from build123d import *

# Parameters (mm, degrees)
BOSS_EXTRUDE1_REACH = 15.24
SKETCH2_R           = 4.7625


with BuildPart() as part:
    # Sketch1 → Revolve1 (revolve)
    with BuildSketch(Plane(origin=(0, 0, 0), x_dir=(0, 0, -1), z_dir=(1, 0, 0)), mode=Mode.PRIVATE) as revolve1_sk:
        Polygon((0, 4.7625), (-7.1628, 4.7625), (-7.1628, 5.55625), (-3.90525, 5.55625), (-1.5875, 7.874), (0, 7.874), align=None)
    revolve(revolve1_sk.sketch.rotate(Axis((0, 0, 0), (0, 0, 1)), 90), axis=Axis((0, 0, 0), (0, 0, 1)))

    # Boss-Extrude1: up to this cone (the profile starts outside it)
    boss_extrude1_end = Plane(origin=(0, 0, 7.1628), z_dir=(0, 0, -1)).offset(-2.298699) * Cone(1e-06, 20.3374, 20.337399, align=(Align.CENTER, Align.CENTER, Align.MIN), mode=Mode.PRIVATE)
    # Sketch2 → Boss-Extrude1 (add, up to the surface)
    with BuildSketch(Plane.XY.offset(7.1628), mode=Mode.PRIVATE) as boss_extrude1_sk1:
        Polygon((-3.207902433, 5.55625), (-6.415804866, 0), (-3.207902433, -5.55625), (3.207902433, -5.55625), (6.415804866, 0), (3.207902433, 5.55625), align=None)
        with Locations(Location((0, 0, 0), (0, 0, 180))):
            Circle(SKETCH2_R, mode=Mode.SUBTRACT)
    boss_extrude1_tool1 = extrude(boss_extrude1_sk1.sketch, amount=-BOSS_EXTRUDE1_REACH, mode=Mode.PRIVATE) - boss_extrude1_end
    add(boss_extrude1_tool1.solids().sort_by_distance((-4.664849, 2.693252, 7.1628))[0])


solid = part.part
Model file for the job. Use its own axes, mm. A direction names the side the tool comes from. Give positions to 0.01 mm unless a question says otherwise; leave off trailing zeros. Loops run counter-clockwise (first coordinate to the right, second up) from the corner with the lowest first, then second, coordinate; pieces in that order, holes last.
1) Wall check: line 1 (Y direction, x = -3.25, z = 2.25); line 2 (Y direction, x = 0, z = 2.5); line 3 (X direction, y = -3.25, z = 4.5). Give the ranges that are in metal, low to high.
2) Saw through at C-C (z = 0.75). Write the cut outline in (x, y) (1 decimal), plus the area to 3 significant figures.
3) Pull direction Y, two halves, no side cores. Call faces 1 (the flat face through (4.8, -2.8, 5.6)), 2 (the flat face through (0, 5.556, 6)), 3 (the cylindrical face through (1.03, 4.65, 3.63)): +Y half, -Y half, draft (parallel to the pull), parting line (faces both ways), or undercut.
4) Tool access for faces 4 (the flat face through (-4.834, -2.739, 5.591)), 5 (the flat face through (4.834, 2.739, 5.591)), 6 (the flat face through (-4.8, 2.8, 5.6)): list every direction of +Z, -Z, +X, -X, +Y, -Y with a clear straight run to the whole face (end or side of a thin tool).
5) Saw through at B-B (x = 0). Write the cut outline in (y, z).
6) Flat gauge pins, fed straight in: pin 1 Ø1 at (x, z) = (-2, 3) entering from -Y; pin 2 Ø3.5 at (x, z) = (-1.5, 5) entering from -Y; pin 3 Ø1 at (x, z) = (-5, 2) entering from -Y. Where does each tip first touch, or does it go through?
7) Saw through at A-A (z = 4.75). Write the cut outline in (x, y) (1 decimal), plus the area to 3 significant figures.
Answer block:
1. line 1: y = -6.44 to -3.48, 3.48 to 6.44
1. line 2: y = -6.96 to -4.76, 4.76 to 6.96
1. line 3: x = -4.54 to -3.48, 3.48 to 4.54
2. outline: circle Ø15.7 at (0, 0); hole circle Ø9.5 at (0, 0)
2. area: 124 mm2
3. face 1: -Y half
3. face 2: +Y half
3. face 3: undercut
4. face 4: +Z, -X, -Y
4. face 5: +Z, +X, +Y
4. face 6: +Z, -X, +Y
5. outline: (-7.87, 0) - (-4.76, 0) - (-4.76, 7.16) - (-5.56, 7.16) - (-5.56, 3.91) - (-7.87, 1.59) - close; (4.76, 0) - (7.87, 0) - (7.87, 1.59) - (5.56, 3.91) - (5.56, 7.16) - (4.76, 7.16) - close
6. pin 1: stops at y = -6.69
6. pin 2: stops at y = -6.07
6. pin 3: stops at y = -6.3
7. outline: (-6.4, 0) - (-3.2, -5.6) - (3.2, -5.6) - (6.4, 0) - (3.2, 5.6) - (-3.2, 5.6) - close; hole circle Ø9.5 at (0, 0)
7. area: 35.7 mm2
